Geometry check sheet. Reference: the model listing, model coordinates, mm. Face numbers are marked on the shaded views. A direction names the side the tool comes from. Round coordinates to 2 decimals unless told otherwise and drop trailing zeros. Order: outer loops, then holes, each group sorted by start corner. A loop starts at its lowest first (then second) coordinate and runs counter-clockwise, first axis right, second up. Notation, with made-up numbers: (19, 43.5) - (45, 43.5) arc R28 ccw to (45, 61.5) - close; hole circle Ø4 at (-33, 66). An arc over 180 degrees is marked (long way). Return JSON: item names as keys, results as strings. Group by question number.
Q1. Gauge pin test, flat ends, axial feed: pin 1 Ø12 at (x, z) = (177.5, 7.5) entering from -Y; pin 2 Ø4.5 at (x, y) = (161.42, 182.34) entering from +Z; pin 3 Ø1 at (x, z) = (178, 2.5) entering from +Y; pin 4 Ø12 at (x, z) = (258, 19) entering from +Y. Record the tip position at first contact, or that the pin passes through.
Q2. Material ranges on line 1 along Z through (x, y) = (210, 179.5); line 2 along Y through (x, z) = (220, 16); line 3 along Y through (x, z) = (248, 9.5), recorded low to high.
Q3. Tool access check on the marked faces 4 and 5. Record the directions out of +Z, -Z, +X, -X, +Y, -Y that give a thin tool (end or side, any length) a straight path to the whole face; none if there is none.
Q4. Sectioned sample at A-A, the plane x = 271. Record the cut outline in (y, z), then the cut area to 3 significant figures.
Q5. Sectioned sample at B-B, the plane y = 190. Record the cut outline in (x, z).
Q6. Sectioned sample at C-C, the plane z = 12.75. Record the cut outline in (x, y).
Q7. Draft check along Z on the marked faces 1, 2 and 3. Enter one of: pulls with the +Z half, pulls with the -Z half, needs draft (parallel to the pull), parting line crosses it, or undercut.
```python
from build123d import *

# Parameters (mm, degrees)
SKETCH1_R                     = 1.5
SKETCH1_R_2                   = 2
BASE_FLANGE1_DEPTH            = 1.4
EDGE_FLANGE1_STRIP_W          = 8.6
EDGE_FLANGE1_STRIP_H          = 1.4
EDGE_FLANGE1_STRIP_CUT_DEPTH  = 95.413569059
EDGE_FLANGE1_RELIEF_W         = 9.3
EDGE_FLANGE1_RELIEF_H         = 0.7
EDGE_FLANGE1_RELIEF_CUT_DEPTH = 1.4
EDGE_FLANGE1_DEPTH            = 95.413569059


# Sheet-metal steps are written as plain solids
with BuildPart() as part:
    # Sketch1 → Base-Flange1 (new body)
    with BuildSketch(Plane.XY):
        with BuildLine():
            Line((170.912926542, 175.40661908), (266.125044601, 169.209705713))
            ThreePointArc((266.125044601, 169.209705713), (267.39344589, 169.561157821), (268.168771741, 170.624750901))
            Line((268.168771741, 170.624750901), (275.774482778, 195.689745971))
            ThreePointArc((275.774482778, 195.689745971), (276.665177338, 196.827499007), (278.089902914, 197.068280651))
            Line((278.089902914, 197.068280651), (286.893064256, 195.263905966))
            ThreePointArc((286.893064256, 195.263905966), (288.317789833, 195.50468761), (289.208484393, 196.642440646))
            Line((289.208484393, 196.642440646), (291.575051406, 204.441578719))
            ThreePointArc((291.575051406, 204.441578719), (291.26768584, 206.213641138), (289.661220117, 207.02231084))
            Line((289.661220117, 207.02231084), (276.272582238, 207.02231084))
            ThreePointArc((276.272582238, 207.02231084), (275.645401821, 206.921427667), (275.081493354, 206.628955565))
            Line((275.081493354, 206.628955565), (256.422617181, 192.796164997))
            ThreePointArc((256.422617181, 192.796164997), (255.8954918, 192.516238104), (255.30923711, 192.404319956))
            Line((255.30923711, 192.404319956), (161.178140888, 188.744148243))
            ThreePointArc((161.178140888, 188.744148243), (155.343352432, 183.233583314), (160.019332793, 176.710831608))
            Line((160.019332793, 176.710831608), (170.912926542, 175.40661908))
        make_face()
        with Locations((287.294653103, 201.429207007)):
            Circle(SKETCH1_R, mode=Mode.SUBTRACT)
        with Locations((161.415148292, 182.342793615)):
            Circle(SKETCH1_R_2, mode=Mode.SUBTRACT)
        with BuildLine():
            Line((261.718420137, 179.964788264), (262.260552067, 181.889909811))
            ThreePointArc((262.260552067, 181.889909811), (264.234354849, 182.996301504), (265.340746542, 181.022498723))
            Line((265.340746542, 181.022498723), (264.798614613, 179.097377176))
            ThreePointArc((264.798614613, 179.097377176), (262.824811831, 177.990985482), (261.718420137, 179.964788264))
        make_face(mode=Mode.SUBTRACT)
    extrude(amount=-BASE_FLANGE1_DEPTH)

    # Edge-Flange1 strip (across the edge) → Edge-Flange1 strip cut (cut)
    with BuildSketch(Plane(origin=(170.912926542, 175.40661908, 0), x_dir=(0.06494792541912509, 0.9978886546021816, 3.4914813388431334e-15), z_dir=(0.9978886546021816, -0.06494792541912509, 0))):
        with Locations((-2.8, -0.7)):
            Rectangle(EDGE_FLANGE1_STRIP_W, EDGE_FLANGE1_STRIP_H)
    extrude(amount=EDGE_FLANGE1_STRIP_CUT_DEPTH, mode=Mode.SUBTRACT)

    # Edge-Flange1 relief (on the sheet) → Edge-Flange1 relief cut (cut)
    with BuildSketch(Plane(origin=(171.01034843, 176.903452062, 0), x_dir=(0.06494792541912509, 0.9978886546021816, 6.982962677686267e-15), z_dir=(0, 0, 1))):
        with Locations((-3.95, 0.35)):
            Rectangle(EDGE_FLANGE1_RELIEF_W, EDGE_FLANGE1_RELIEF_H)
        with Locations((-3.95, -95.763569059)):
            Rectangle(EDGE_FLANGE1_RELIEF_W, EDGE_FLANGE1_RELIEF_H)
    extrude(amount=-EDGE_FLANGE1_RELIEF_CUT_DEPTH, mode=Mode.SUBTRACT)

    # Edge-Flange1 section (across the edge) → Edge-Flange1 (add)
    with BuildSketch(Plane(origin=(170.912926542, 175.40661908, 0), x_dir=(0.06494792541912509, 0.9978886546021816, 3.4914813388431334e-15), z_dir=(0.9978886546021816, -0.06494792541912509, 0))):
        with BuildLine():
            Line((-1.4, 1.5), (-1.4, 11))
            Line((-1.4, 11), (0, 11))
            Line((0, 11), (0, 1.5))
            ThreePointArc((0, 1.5), (0.439339828, 0.439339828), (1.5, 0))
            Line((1.5, 0), (1.5, -1.4))
            ThreePointArc((1.5, -1.4), (-0.550609665, -0.550609665), (-1.4, 1.5))
        make_face()
    extrude(amount=EDGE_FLANGE1_DEPTH)

    # Mirror1: part across plane


with BuildPart() as part_1:
    add(part.part)
    add(part.part.mirror(Plane(origin=(170.821999446, 174.009574964, 11), x_dir=(1, 0, 0), z_dir=(0, 0, -1))))


solid = part_1.part
```
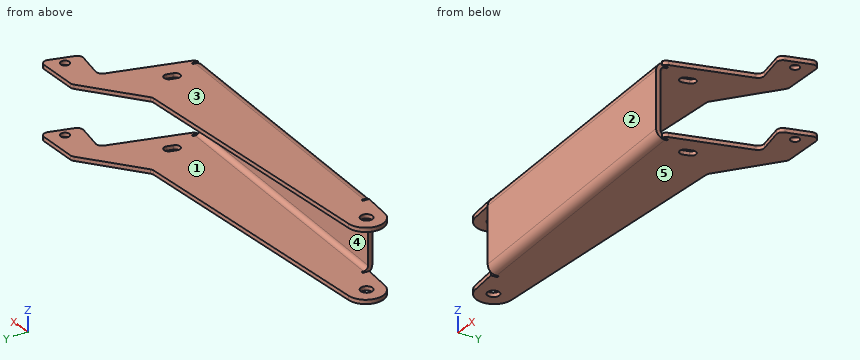
Reply:
{
 "1": {"pin 1": "y = 173.18", "pin 2": "z = 23.4", "pin 3": "y = 174.98", "pin 4": "y = 197.82"},
 "2": {"line 1": "-1.4 to 0, 22 to 23.4", "line 2": "170.81 to 172.21", "line 3": "168.99 to 170.39"},
 "3": {"face 4": "+X, +Y", "face 5": "-Z, +X, -X, +Y, -Y"},
 "4": {"outline": "(179.96, -1.4) - (203.6, -1.4) - (203.6, 0) - (179.96, 0) - close; (179.96, 22) - (203.6, 22) - (203.6, 23.4) - (179.96, 23.4) - close", "area": "66.2 mm^2"},
 "5": {"outline": "(193.48, -1.4) - (274.05, -1.4) - (274.05, 0) - (193.48, 0) - close; (193.48, 22) - (274.05, 22) - (274.05, 23.4) - (193.48, 23.4) - close"},
 "6": {"outline": "(170.82, 174.01) - (266.03, 167.81) - (266.13, 169.21) - (170.91, 175.41) - close"},
 "7": {"face 1": "undercut", "face 2": "needs draft", "face 3": "pulls with the +Z half"}
}
